```python
from build123d import *

# Parameters (mm, degrees)
BOSS_EXTRU_1_DEPTH                  = 2
BOSS_EXTRU_2_DEPTH                  = 28
ENL_V_MAT_EXTRU_1_DEPTH             = 28
BOSS_EXTRU_3_DEPTH                  = 22
BOSS_EXTRU_4_DEPTH                  = 6
BOSS_EXTRU_5_DEPTH                  = 22
BOSS_EXTRU_6_DEPTH                  = 6
BOSS_EXTRU_7_DEPTH                  = 22
BOSS_EXTRU_8_DEPTH                  = 6
BOSS_EXTRU_9_DEPTH                  = 22
BOSS_EXTRU_10_DEPTH                 = 6
ENL_V_MAT_EXTRU_2_REACH             = 116.632
ESQUISSE12_W                        = 12
ESQUISSE12_H                        = 12
ESQUISSE13_W                        = 12
ESQUISSE13_H                        = 12
ENL_V_MAT_EXTRU_3_DEPTH             = 115.63237734
D_POUILLE1_ANGLE                    = 1
DIAM_TRE_DU_PER_AGE_6_0_6_1_D       = 6
DIAM_TRE_DU_PER_AGE_6_0_6_1_DEPTH   = 30
DIAM_TRE_DU_PER_AGE_1_8_1_8_1_D     = 1.8
DIAM_TRE_DU_PER_AGE_1_8_1_8_1_DEPTH = 7
PER_AGE1_D                          = 2.65
PER_AGE1_DEPTH                      = 8
CONG_1_R                            = 1
CONG_2_R                            = 10


with BuildPart() as part:
    # Esquisse1 → Boss.-Extru.1 (new body)
    with BuildSketch(Plane.XZ.offset(-7.6)):
        with BuildLine():
            Line((63.019312785, 0), (43.183766285, 28.246822547))
            ThreePointArc((43.183766285, 28.246822547), (39.611495122, 31.373224484), (35, 32.5))
            Line((35, 32.5), (-35, 32.5))
            ThreePointArc((-35, 32.5), (-39.611495122, 31.373224484), (-43.183766285, 28.246822547))
            Line((-43.183766285, 28.246822547), (-63.019312785, 0))
            Line((-63.019312785, 0), (-43.183766285, -28.246822547))
            ThreePointArc((-43.183766285, -28.246822547), (-39.611495122, -31.373224484), (-35, -32.5))
            Line((-35, -32.5), (35, -32.5))
            ThreePointArc((35, -32.5), (39.611495122, -31.373224484), (43.183766285, -28.246822547))
            Line((43.183766285, -28.246822547), (63.019312785, 0))
        make_face()
    extrude(amount=-BOSS_EXTRU_1_DEPTH)

    # Esquisse2 → Boss.-Extru.2 (add)
    with BuildSketch(Plane.XZ.offset(-7.6)):
        with BuildLine():
            Line((-45, -22.5), (-45, 22.5))
            ThreePointArc((-45, 22.5), (-42.071067812, 29.571067812), (-35, 32.5))
            Line((-35, 32.5), (35, 32.5))
            ThreePointArc((35, 32.5), (42.071067812, 29.571067812), (45, 22.5))
            Line((45, 22.5), (45, -22.5))
            ThreePointArc((45, -22.5), (42.071067812, -29.571067812), (35, -32.5))
            Line((35, -32.5), (-35, -32.5))
            ThreePointArc((-35, -32.5), (-42.071067812, -29.571067812), (-45, -22.5))
        make_face()
    extrude(amount=BOSS_EXTRU_2_DEPTH)

    # Esquisse3 → Enlèv. mat.-Extru.1 (cut)
    with BuildSketch(Plane.XZ.offset(20.4)):
        with BuildLine():
            Line((43, -22.5), (43, 22.5))
            ThreePointArc((43, 22.5), (40.656854249, 28.156854249), (35, 30.5))
            Line((35, 30.5), (-35, 30.5))
            ThreePointArc((-35, 30.5), (-40.656854249, 28.156854249), (-43, 22.5))
            Line((-43, 22.5), (-43, -22.5))
            ThreePointArc((-43, -22.5), (-40.656854249, -28.156854249), (-35, -30.5))
            Line((-35, -30.5), (35, -30.5))
            ThreePointArc((35, -30.5), (40.656854249, -28.156854249), (43, -22.5))
        make_face()
    extrude(amount=-ENL_V_MAT_EXTRU_1_DEPTH, mode=Mode.SUBTRACT)

    # Esquisse4 → Boss.-Extru.3 (add)
    with BuildSketch(Plane.XZ.offset(-7.6)):
        with BuildLine():
            Line((42.708099244, -15.5), (43, -15.5))
            Line((43, -15.5), (43, -18.5))
            Line((43, -18.5), (42.708099244, -18.5))
            ThreePointArc((42.708099244, -18.5), (35, -17), (42.708099244, -15.5))
        make_face()
    extrude(amount=BOSS_EXTRU_3_DEPTH)

    # Esquisse5 → Boss.-Extru.4 (add)
    with BuildSketch(Plane.XZ.offset(-7.6)):
        with BuildLine():
            Line((34.492820127, -19.515715167), (35.346896814, -18.629367089))
            ThreePointArc((35.346896814, -18.629367089), (36.224495368, -19.880377412), (37.507179873, -20.710995563))
            Line((37.507179873, -20.710995563), (36.653103186, -21.597343641))
            ThreePointArc((36.653103186, -21.597343641), (30.224495368, -26.107088143), (34.492820127, -19.515715167))
        make_face()
    extrude(amount=BOSS_EXTRU_4_DEPTH)

    # Esquisse6 → Boss.-Extru.5 (add)
    with BuildSketch(Plane.XZ.offset(-7.6)):
        with BuildLine():
            Line((-42.708099244, -18.5), (-43, -18.5))
            Line((-43, -18.5), (-43, -15.5))
            Line((-43, -15.5), (-42.708099244, -15.5))
            ThreePointArc((-42.708099244, -15.5), (-35, -17), (-42.708099244, -18.5))
        make_face()
    extrude(amount=BOSS_EXTRU_5_DEPTH)

    # Esquisse7 → Boss.-Extru.6 (add)
    with BuildSketch(Plane.XZ.offset(-7.6)):
        with BuildLine():
            Line((-36.682682292, -21.438638051), (-37.438638051, -20.682682292))
            ThreePointArc((-37.438638051, -20.682682292), (-36.171572875, -19.828427125), (-35.317317708, -18.561361949))
            Line((-35.317317708, -18.561361949), (-34.561361949, -19.317317708))
            ThreePointArc((-34.561361949, -19.317317708), (-30.171572875, -25.828427125), (-36.682682292, -21.438638051))
        make_face()
    extrude(amount=BOSS_EXTRU_6_DEPTH)

    # Esquisse8 → Boss.-Extru.7 (add)
    with BuildSketch(Plane.XZ.offset(-7.6)):
        with BuildLine():
            Line((42.708099244, 18.5), (43, 18.5))
            Line((43, 18.5), (43, 15.5))
            Line((43, 15.5), (42.708099244, 15.5))
            ThreePointArc((42.708099244, 15.5), (35, 17), (42.708099244, 18.5))
        make_face()
    extrude(amount=BOSS_EXTRU_7_DEPTH)

    # Esquisse9 → Boss.-Extru.8 (add)
    with BuildSketch(Plane.XZ.offset(-7.6)):
        with BuildLine():
            Line((36.682682292, 21.438638051), (37.438638051, 20.682682292))
            ThreePointArc((37.438638051, 20.682682292), (36.171572875, 19.828427125), (35.317317708, 18.561361949))
            Line((35.317317708, 18.561361949), (34.561361949, 19.317317708))
            ThreePointArc((34.561361949, 19.317317708), (30.171572875, 25.828427125), (36.682682292, 21.438638051))
        make_face()
    extrude(amount=BOSS_EXTRU_8_DEPTH)

    # Esquisse10 → Boss.-Extru.9 (add)
    with BuildSketch(Plane.XZ.offset(-7.6)):
        with BuildLine():
            Line((-42.708099244, 15.5), (-43, 15.5))
            Line((-43, 15.5), (-43, 18.5))
            Line((-43, 18.5), (-42.708099244, 18.5))
            ThreePointArc((-42.708099244, 18.5), (-35, 17), (-42.708099244, 15.5))
        make_face()
    extrude(amount=BOSS_EXTRU_9_DEPTH)

    # Esquisse11 → Boss.-Extru.10 (add)
    with BuildSketch(Plane.XZ.offset(-7.6)):
        with BuildLine():
            Line((-34.561361949, 19.317317708), (-35.317317708, 18.561361949))
            ThreePointArc((-35.317317708, 18.561361949), (-36.171572875, 19.828427125), (-37.438638051, 20.682682292))
            Line((-37.438638051, 20.682682292), (-36.682682292, 21.438638051))
            ThreePointArc((-36.682682292, 21.438638051), (-30.171572875, 25.828427125), (-34.561361949, 19.317317708))
        make_face()
    extrude(amount=BOSS_EXTRU_10_DEPTH)

    # Esquisse12 → Enlèv. mat.-Extru.2 (cut, up to next)
    with BuildSketch(Plane.ZY.offset(45), mode=Mode.PRIVATE) as enl_v_mat_extru_2_sk1:
        with Locations((0, -5.4)):
            Rectangle(ESQUISSE12_W, ESQUISSE12_H)
    enl_v_mat_extru_2_tool1 = extrude(enl_v_mat_extru_2_sk1.sketch, amount=-ENL_V_MAT_EXTRU_2_REACH, mode=Mode.PRIVATE) & part.part
    add(enl_v_mat_extru_2_tool1.solids().sort_by_distance((-45, -5.4, 0))[0], mode=Mode.SUBTRACT)

    # Esquisse13 → Enlèv. mat.-Extru.3 (cut, through all)
    with BuildSketch(Plane(origin=(45, 0, 0), x_dir=(0, 0, -1), z_dir=(1, 0, 0))):
        with Locations((0, -5.4)):
            Rectangle(ESQUISSE13_W, ESQUISSE13_H)
    extrude(amount=-ENL_V_MAT_EXTRU_3_DEPTH, mode=Mode.SUBTRACT)

    # Dépouille1
    d_pouille1_faces = [part.faces().sort_by_distance(p)[0] for p in [
        (-35, -3.4, 17),
        (35, -3.4, 17),
        (35, -3.4, -17),
        (-35, -3.4, -17),
    ]]
    draft(d_pouille1_faces, Plane(origin=(35, 7.6, -22.5), x_dir=(0, 0, -1), z_dir=(0, -1, 0)), D_POUILLE1_ANGLE)

    # Diamètre du perçage Ø6.0 (6)1
    with Locations(Plane(origin=(0, 9.6, 0), x_dir=(1, 0, 0), z_dir=(0, 1, 0))):
        with Locations((-50.8, 0), (50.8, 0)):
            Hole(DIAM_TRE_DU_PER_AGE_6_0_6_1_D / 2, depth=DIAM_TRE_DU_PER_AGE_6_0_6_1_DEPTH)

    # Diamètre du perçage Ø1.8 (1.8)1
    with Locations(Plane(origin=(0, 1.6, 0), x_dir=(-1, 0, 0), z_dir=(0, -1, 0))):
        with Locations((33, -23), (-33, -23), (-33, 23.22671073), (33, 23)):
            Hole(DIAM_TRE_DU_PER_AGE_1_8_1_8_1_D / 2, depth=DIAM_TRE_DU_PER_AGE_1_8_1_8_1_DEPTH)

    # Perçage1
    with Locations(Plane(origin=(0, -14.4, 0), x_dir=(-1, 0, 0), z_dir=(0, -1, 0))):
        with Locations((-39, 17), (-39, -17), (39, 17), (39, -17)):
            Hole(PER_AGE1_D / 2, depth=PER_AGE1_DEPTH)

    # Congé1
    cong_1_edges = [part.edges().sort_by_distance(p)[0] for p in [
        (-44, -11.4, -6),
        (-44, 0.6, -6),
        (-44, 0.6, 6),
        (-44, -11.4, 6),
        (44, -11.4, -6),
        (44, 0.6, 6),
        (44, 0.6, -6),
        (44, -11.4, 6),
    ]]
    fillet(cong_1_edges, radius=CONG_1_R)

    # Congé2
    cong_2_edges = [part.edges().sort_by_distance(p)[0] for p in [
        (-63.019312785, 8.6, 0),
        (63.019312785, 8.6, 0),
    ]]
    fillet(cong_2_edges, radius=CONG_2_R)


solid = part.part
```
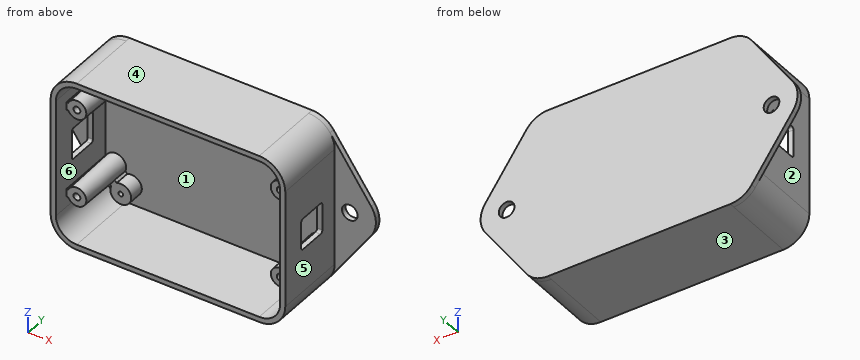
Source: CAD feature listing. Evaluate the final solid. Frame: model axes, mm. Face numbers are marked on the shaded views. A direction names the side the tool comes from. Coordinates: 2 decimals unless noted, no trailing zeros. Loops run counter-clockwise (first coordinate to the right, second up) from the corner with the lowest first, then second, coordinate; pieces in that order, holes last. Notation, with made-up numbers: M 8.5,10 L 34.5,10 A16 cw 34.5,14 Z; hole C -2,9.25 d8. An arc over 180 degrees is marked long. Put each result on its own line as item: value. Start each with the question number.
1) Pull-direction query (Z, two-part tool) for the marked faces 1, 2 and 3; classes: pulls with the +Z half, pulls with the -Z half, needs draft (parallel to the pull), parting line crosses it, or undercut.
2) Cut plane A-A on x = 26. Return the cut outline in (y, z).
3) Ray query, L1, parallel to X at y = 4.75, z = -3.5; L2, parallel to Z at x = -33, y = 7; L3, parallel to Z at x = -39, y = -7.75 (3 decimals). Return the intervals inside material, ascending. Write a range as from..to.
4) Cut plane B-B on x = 50.8. Return the cut outline in (y, z).
5) Reachability of the marked faces 4, 5 and 6 from +Z, -Z, +X, -X, +Y, -Y: full face, straight path, thin tool, end or side. Return the list, or none.
6) Contact query for flat-ended pins moving along their axis: pin 1 Ø2.5 at (x, z) = (39, -17) entering from -Y; pin 2 Ø3 at (y, z) = (0, 1.5) entering from -X; pin 3 Ø2 at (x, z) = (37.5, -16.5) entering from -Y. Output: stop coordinate, or through.
The answers:
1. face 1: undercut
1. face 2: needs draft
1. face 3: pulls with the -Z half
2. outline: M -20.4,-32.5 L 9.6,-32.5 L 9.6,32.5 L -20.4,32.5 L -20.4,30.5 L 7.6,30.5 L 7.6,-30.5 L -20.4,-30.5 Z
3. L1: x = -45..-43, 43..45
3. L2: z = -32.5..-30.5, -27..-23.9, -22.1..-19, 19..22.1, 23.9..27, 30.5..32.5
3. L3: z = -31.665..-29.428, -20.732..-18.325, -15.675..-13.268, 13.268..15.675, 18.325..20.732, 29.428..31.665
4. outline: M 7.6,-17.4 L 9.6,-17.4 L 9.6,-3 L 7.6,-3 Z; M 7.6,3 L 9.6,3 L 9.6,17.4 L 7.6,17.4 Z
5. face 4: +Z, +X, -X, +Y, -Y
5. face 5: +Z, -Z, +X, -Y
5. face 6: -Y
6. pin 1: stops at y = -6.4
6. pin 2: stops at x = -45
6. pin 3: stops at y = -14.4
